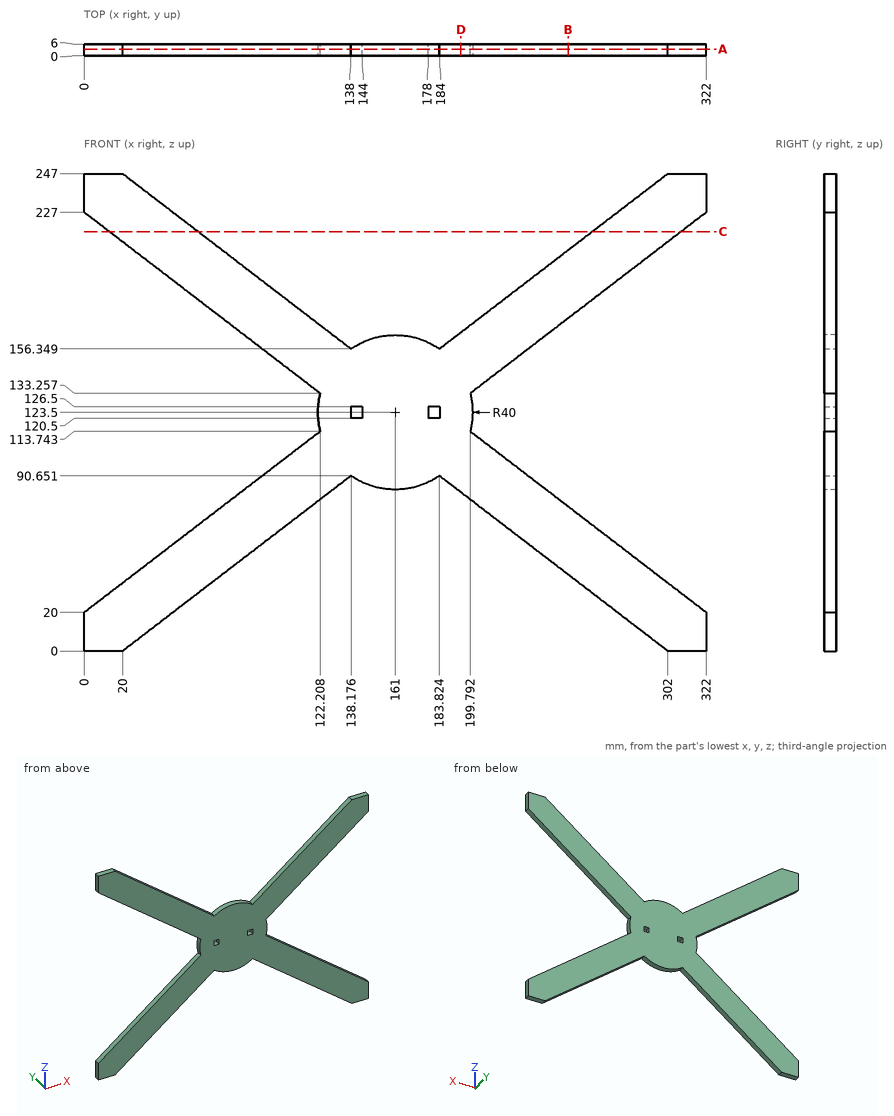
Study the drawing (mm; zero at the part's minimum x, y, z) and answer. Round coordinates to 2 decimals unless told otherwise and drop trailing zeros. Loops run counter-clockwise (first coordinate to the right, second up) from the corner with the lowest first, then second, coordinate; pieces in that order, holes last. Notation, with made-up numbers: (54.5, 27.25) -> (109.5, 27.25) arc R16 cw to (109.5, 40.25) -> close; hole circle Ø6 at (55.25, 21.25). An arc over 180 degrees is marked (long way). Write each question's results on one line, items separated by ' | '. Start each with the question number.
1. Find the intervals of material crossed by probe 1 along Z at (x, y) = (299, 1.45) (1 decimal); probe 2 along Z at (x, y) = (296, 5.3) (1 decimal); probe 3 along X at (y, z) = (3.55, 183.5) (1 decimal), in increasing order. Write a range as from..to.
2. Section D-D (x = 195) is taken. Determine the outline of the cut face in (y, z).
3. Section A-A (y = 3.4) is taken. Determine the outline of the cut face in (x, z).
4. Section C-C (z = 217) is taken. Determine the outline of the cut face in (x, y).
5. Section B-B (x = 250.5) is taken. Determine the outline of the cut face in (y, z) (1 decimal), plus the area to 3 significant figures.
6. Given pin 1 Ø1.5 at (x, y) = (151.5, 1.5) entering from -Z; pin 2 Ø3 at (x, y) = (182.5, 3) entering from -Z; pin 3 Ø3 at (y, z) = (2.5, 124) entering from +X, each flat-ended and moving along its own axis, determine where each tip first touches the part or whether it passes through.
Evaluation:
1) probe 1: z = 2.3..37.6, 209.4..244.7 | probe 2: z = 4.6..39.9, 207.1..242.4 | probe 3: x = 56.7..102.8, 219.2..265.3
2) outline: (0, 82.08) -> (6, 82.08) -> (6, 164.92) -> (0, 164.92) -> close
3) outline: (0, 0) -> (20, 0) -> (138.18, 90.65) arc R40 ccw to (183.82, 90.65) -> (302, 0) -> (322, 0) -> (322, 20) -> (199.79, 113.74) arc R40 ccw to (199.79, 133.26) -> (322, 227) -> (322, 247) -> (302, 247) -> (183.82, 156.35) arc R40 ccw to (138.18, 156.35) -> (20, 247) -> (0, 247) -> (0, 227) -> (122.21, 133.26) arc R40 ccw to (122.21, 113.74) -> (0, 20) -> close; hole (138, 120.5) -> (144, 120.5) -> (144, 126.5) -> (138, 126.5) -> close; hole (178, 120.5) -> (184, 120.5) -> (184, 126.5) -> (178, 126.5) -> close
4) outline: (13.04, 0) -> (59.11, 0) -> (59.11, 6) -> (13.04, 6) -> close; (262.89, 0) -> (308.96, 0) -> (308.96, 6) -> (262.89, 6) -> close
5) outline: (0, 39.5) -> (6, 39.5) -> (6, 74.8) -> (0, 74.8) -> close; (0, 172.2) -> (6, 172.2) -> (6, 207.5) -> (0, 207.5) -> close | area: 424 mm2
6) pin 1: stops at z = 84.47 | pin 2: stops at z = 88.86 | pin 3: stops at x = 201
